```python
from build123d import *

# Parameters (mm, degrees)
BOSS_EXTRUDE1_DEPTH = 206.375
FILLET1_R           = 0.889


with BuildPart() as part:
    # Sketch1 → Boss-Extrude1 (new body)
    with BuildSketch(Plane.XY):
        with BuildLine():
            Line((-0.396875, 3.175), (0, 0))
            Line((0, 0), (-2.38125, 0))
            Line((-2.38125, 0), (-2.38125, 1.5875))
            ThreePointArc((-2.38125, 1.5875), (-6.310112, 3.214888), (-7.9375, 7.14375))
            Line((-7.9375, 7.14375), (-7.9375, 8.73125))
            Line((-7.9375, 8.73125), (-9.525, 8.73125))
            Line((-9.525, 8.73125), (-9.525, 14.2875))
            Line((-9.525, 14.2875), (-1.238157, 14.2875))
            Line((-1.238157, 14.2875), (-0.887649, 20.6375))
            Line((-0.887649, 20.6375), (0, 20.588503))
            Line((0, 20.588503), (-0.396875, 13.3985))
            Line((-0.396875, 13.3985), (-8.636, 13.3985))
            Line((-8.636, 13.3985), (-8.636, 9.62025))
            Line((-8.636, 9.62025), (-7.0485, 9.62025))
            Line((-7.0485, 9.62025), (-7.0485, 7.14375))
            ThreePointArc((-7.0485, 7.14375), (-5.350597, 3.542888), (-1.49225, 2.561949))
            Line((-1.49225, 2.561949), (-1.49225, 0.889))
            Line((-1.49225, 0.889), (-1.007043, 0.889))
            Line((-1.007043, 0.889), (-1.27901, 3.064733))
            Line((-1.27901, 3.064733), (-0.396875, 3.175))
        make_face()
    extrude(amount=-BOSS_EXTRUDE1_DEPTH)

    # Fillet1
    fillet1_edges = [part.edges().sort_by_distance(p)[0] for p in [
        (-2.38125, 0, -103.1875),
        (-9.525, 8.73125, -103.1875),
        (-9.525, 14.2875, -103.1875),
        (-0.396875, 13.3985, -103.1875),
        (-7.0485, 9.62025, -103.1875),
        (-1.49225, 2.561949, -103.1875),
    ]]
    fillet(fillet1_edges, radius=FILLET1_R)


solid = part.part
```
For this review, take the finished solid that the model builds, in its own axes (mm). A direction names the side the tool comes from. Give positions to 0.01 mm unless a question says otherwise; leave off trailing zeros. Order: outer loops, then holes, each group sorted by start corner. A loop starts at its lowest first (then second) coordinate and runs counter-clockwise, first axis right, second up.
1) The part is to be moulded in two halves that separate along Y. For faces 1 (the face through (-0.2, 1.6, -101.7)), 2 (the face through (-6.267, 3.172, -101.743)), 3 (the face through (-1.065, 17.418, -101.743)), 4 (the face through (-5, 13.398, -102)), say which applies: released by +Y, released by -Y, zero draft, split by the parting line, or undercut.
2) Insertion check: pin 1 (3 mm diameter, centred on x = -8, z = -110.5, fed in from -Y); pin 2 (3.5 mm diameter, centred on x = -5, z = -127, fed in from -Y); pin 3 (0.6 mm diameter, centred on x = -8.5, z = -95, fed in from +Y). Each pin has a flat end and moves straight along its axis. Give the tip position at first contact, or say it passes through.
3) Take a section at A-A (x = -4.75). Give the boundary of the cut face in (y, z) (1 decimal), then the cut area to 3 significant figures.
4) Take a section at D-D (y = 17). Give the boundary of the cut face in (x, z) (3 decimals), then the cut area to 3 significant figures.
5) Take a section at C-C (y = 5). Give the boundary of the cut face in (x, z) (3 decimals), then the cut area to 3 significant figures.
6) For faces 5 (the face through (-9.525, 11, -102)), 6 (the face through (-0.173, 17.458, -101.743)), 7 (the face through (-5, 14.288, -102)), 8 (the face through (-7.21, 8.84, 0)), 9 (the face through (-5.72, 3.88, -101.74)), list the 3-axis set-ups (+Z, -Z, +X, -X, +Y, -Y) from which the entire face can be reached by the end or side of a thin tool; tool diameter is ignored.
7) Wall thickness on line 1 (Y direction, x = -8.5, z = -111); line 2 (X direction, y = 11.25, z = -167) (3 decimals); line 3 (Y direction, x = -3.75, z = -22): over which ranges is each line inside the solid? List them lowest first.
8) Take a section at B-B (z = -177.5). Give the boundary of the cut face in (x, y) (1 decimal).
Derived:
1. face 1: undercut
1. face 2: released by -Y
1. face 3: released by +Y
1. face 4: undercut
2. pin 1: stops at y = 3.41
2. pin 2: stops at y = 1.66
2. pin 3: stops at y = 14.29
3. outline: (2.1, -206.4) - (3.1, -206.4) - (3.1, 0) - (2.1, 0) - close; (13.4, -206.4) - (14.3, -206.4) - (14.3, 0) - (13.4, 0) - close
3. area: 391 mm2
4. outline: (-1.088, -206.375) - (-0.198, -206.375) - (-0.198, 0) - (-1.088, 0) - close
4. area: 184 mm2
5. outline: (-7.507, -206.375) - (-6.527, -206.375) - (-6.527, 0) - (-7.507, 0) - close
5. area: 202 mm2
6. face 5: +Z, -Z, -X, +Y, -Y
6. face 6: +Z, -Z, +X
6. face 7: +Z, -Z, -X, +Y
6. face 8: +Z, +X, -X, +Y, -Y
6. face 9: +Z, -Z
7. line 1: y = 8.73 to 9.62, 13.4 to 14.29
7. line 2: x = -9.525 to -8.636
7. line 3: y = 1.76 to 2.68, 13.4 to 14.29
8. outline: (-9.5, 9.6) arc R0.9 ccw to (-8.6, 8.7) - (-7.9, 8.7) - (-7.9, 7.1) arc R5.6 ccw to (-2.4, 1.6) - (-2.4, 0.9) arc R0.9 ccw to (-1.5, 0) - (0, 0) - (-0.4, 3.2) - (-1.3, 3.1) - (-1, 0.9) - (-1.5, 0.9) - (-1.5, 1.6) arc R0.9 ccw to (-2.4, 2.5) arc R4.7 cw to (-7, 7.1) - (-7, 8.7) arc R0.9 ccw to (-7.9, 9.6) - (-8.6, 9.6) - (-8.6, 13.4) - (-1.2, 13.4) arc R0.9 ccw to (-0.4, 14.2) - (0, 20.6) - (-0.9, 20.6) - (-1.2, 14.3) - (-8.6, 14.3) arc R0.9 ccw to (-9.5, 13.4) - close
